from build123d import *
from build123d.topology import SkipClean

# Parameters (mm, degrees)
SKETCH4_R           = 2
BOSS_EXTRUDE1_DEPTH = 140
SKETCH5_W           = 29.5
SKETCH5_H           = 13.79
BOSS_EXTRUDE3_DEPTH = 79.9
SKETCH6_W           = 75.9
SKETCH6_H           = 9.7
CUT_EXTRUDE1_DEPTH  = 27.5
SKETCH7_W           = 23.5
SKETCH7_H           = 26
CUT_EXTRUDE2_DEPTH  = 3
SKETCH8_R           = 2
BOSS_EXTRUDE4_DEPTH = 22.95
SKETCH12_R          = 7
BOSS_EXTRUDE6_DEPTH = 15.01
SKETCH13_R          = 7
BOSS_EXTRUDE7_DEPTH = 4
SKETCH14_R          = 5.5
CUT_EXTRUDE3_DEPTH  = 12


with BuildPart() as part:
    # Sketch4 → Boss-Extrude1 (new body)
    with BuildSketch(Plane(origin=(0, 0, 0), x_dir=(1, 0, 0), z_dir=(0, 1, 0))):
        with Locations(Location((0, -39.95, 0), (0, 0, 270))):
            Circle(SKETCH4_R)
    extrude(amount=BOSS_EXTRUDE1_DEPTH)

    # Sketch5 → Boss-Extrude3 (add)
    with BuildSketch(Plane.XY):
        Rectangle(SKETCH5_W, SKETCH5_H)
    extrude(amount=BOSS_EXTRUDE3_DEPTH)

    # Sketch6 → Cut-Extrude1 (cut)
    with BuildSketch(Plane(origin=(14.75, 0, 0), x_dir=(0, 0, -1), z_dir=(1, 0, 0))):
        with Locations((-39.95, 0)):
            Rectangle(SKETCH6_W, SKETCH6_H)
    extrude(amount=-CUT_EXTRUDE1_DEPTH, mode=Mode.SUBTRACT)

    # Sketch7 → Cut-Extrude2 (cut)
    with BuildSketch(Plane(origin=(0, 6.895, 0), x_dir=(1, 0, 0), z_dir=(0, 1, 0))):
        with Locations((3, -60.9)):
            Rectangle(SKETCH7_W, SKETCH7_H)
    extrude(amount=-CUT_EXTRUDE2_DEPTH, mode=Mode.SUBTRACT)

    # Sketch8 → Boss-Extrude4 (add)
    with SkipClean():  # the faces are left unmerged after this step: merging them gives an invalid solid
        with BuildSketch(Plane.XY.offset(37.95)):
            with Locations((0, 140)):
                Circle(SKETCH8_R)
        extrude(amount=BOSS_EXTRUDE4_DEPTH)

    # Sketch12 → Boss-Extrude6 (add)
    with SkipClean():  # the faces are left unmerged after this step: merging them gives an invalid solid
        with BuildSketch(Plane(origin=(0, 140, 0), x_dir=(1, 0, 0), z_dir=(0, 1, 0))):
            with Locations(Location((0, -60.9, 0), (0, 0, 270))):
                Circle(SKETCH12_R)
        extrude(amount=-BOSS_EXTRUDE6_DEPTH)

    # Sketch13 → Boss-Extrude7 (add)
    with SkipClean():  # the faces are left unmerged after this step: merging them gives an invalid solid
        with BuildSketch(Plane(origin=(0, 140, 0), x_dir=(1, 0, 0), z_dir=(0, 1, 0))):
            with Locations(Location((0, -60.9, 0), (0, 0, 270))):
                Circle(SKETCH13_R)
        extrude(amount=BOSS_EXTRUDE7_DEPTH)

    # Sketch14 → Cut-Extrude3 (cut)
    with SkipClean():  # the faces are left unmerged after this step: merging them gives an invalid solid
        with BuildSketch(Plane.XZ.offset(-124.99)):
            with Locations(Location((0, 60.9, 0), (0, 0, 270))):
                Circle(SKETCH14_R)
        extrude(amount=-CUT_EXTRUDE3_DEPTH, mode=Mode.SUBTRACT)


solid = part.part
For this review, take the finished solid that the model builds, in its own axes (mm). A direction names the side the tool comes from. Give positions to 0.01 mm unless a question says otherwise; leave off trailing zeros. Order: outer loops, then holes, each group sorted by start corner. A loop starts at its lowest first (then second) coordinate and runs counter-clockwise, first axis right, second up. Notation, with made-up numbers: (48, 0.5) -> (100, 0.5) arc R18 cw to (100, 10.5) -> close; hole circle Ø8 at (15, -3). An arc over 180 degrees is marked (long way). Write item = value, one per line.
1) Insertion check: pin 1 (4 mm diameter, centred on x = -1, y = 105.5, fed in from -Z); pin 2 (2 mm diameter, centred on y = 5.5, z = 56, fed in from +X). Each pin has a flat end and moves straight along its axis. Give the tip position at first contact, or say it passes through.
Findings:
pin_1 = 37.95
pin_2 = -8.75
2) We need section B-B, the plane x = -10.5. Give the boundary of the cut face in (y, z) (3 decimals).
Findings:
outline = (-6.895, 0) -> (6.895, 0) -> (6.895, 79.9) -> (-6.895, 79.9) -> close; hole (-4.85, 2) -> (4.85, 2) -> (4.85, 77.9) -> (-4.85, 77.9) -> close
3) We need section D-D, the plane z = 72.5. Give the boundary of the cut face in (x, y) (3 decimals).
Findings:
outline = (-14.75, -6.895) -> (14.75, -6.895) -> (14.75, -4.85) -> (-12.75, -4.85) -> (-12.75, 4.85) -> (-8.75, 4.85) -> (-8.75, 6.895) -> (-14.75, 6.895) -> close
4) To check wall thickness, follow L1, parallel to Y at x = -11, z = 68 (3 decimals); L2, parallel to Z at x = -5, y = 4.5; L3, parallel to Y at x = -2.75, z = 58 (3 decimals). State the ranges of each line that lie inside material, in increasing order. Write a range as from..to.
Findings:
L1 = -6.895..-4.85, 4.85..6.895
L2 = 0..2, 77.9..79.9
L3 = -6.895..-4.85, 136.99..144
5) We need section A-A, the plane z = 60.9. Give the boundary of the cut face in (x, y) (3 decimals), and give its area (3 significant figures).
Findings:
outline = (-14.75, -6.895) -> (14.75, -6.895) -> (14.75, -4.85) -> (-12.75, -4.85) -> (-12.75, 4.85) -> (-8.75, 4.85) -> (-8.75, 6.895) -> (-14.75, 6.895) -> close; (-7, 124.99) -> (-5.5, 124.99) -> (-5.5, 136.99) -> (5.5, 136.99) -> (5.5, 124.99) -> (7, 124.99) -> (7, 144) -> (-7, 144) -> close
area = 226 mm^2
6) Draft analysis for pull direction Z (two halves, no side actions). For faces 4 (the face through (1, 0, 2)), 5 (the face through (14.75, -5, 37)), 6 (the face through (0, 0, 0)), state which applies: pulls with the +Z half, pulls with the -Z half, needs draft (parallel to the pull), parting line crosses it, or undercut.
Findings:
face_4 = undercut
face_5 = needs draft
face_6 = pulls with the -Z half
7) We need section C-C, the plane x = 10.75. Give the boundary of the cut face in (y, z) (3 decimals), and give its area (3 significant figures).
Findings:
outline = (-6.895, 0) -> (6.895, 0) -> (6.895, 47.9) -> (4.85, 47.9) -> (4.85, 2) -> (-4.85, 2) -> (-4.85, 77.9) -> (4.85, 77.9) -> (4.85, 73.9) -> (6.895, 73.9) -> (6.895, 79.9) -> (-6.895, 79.9) -> close
area = 312 mm^2
8) For faces 1 (the face through (-5, 124.99, 64)), 2 (the face through (1.652, 130.906, 55.654)), 3 (the face through (1, 4.85, 32)), list the 3-axis set-ups (+Z, -Z, +X, -X, +Y, -Y) from which the entire face can be reached by the end or side of a thin tool; tool diameter is ignored.
Findings:
face_1 = +Z, +X, -X
face_2 = none
face_3 = +X
